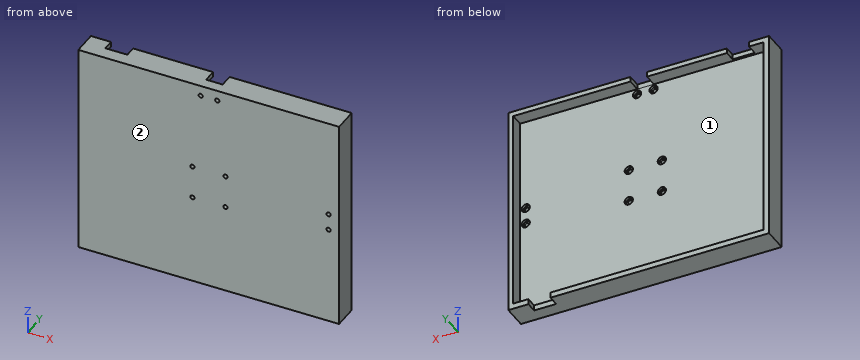
from build123d import *

# Parameters (mm, degrees)
SKETCH2_W                = 236.5
SKETCH2_H                = 193
SKETCH2_W_2              = 227
SKETCH2_H_2              = 183.5
BOSS_EXTRUDE1_DEPTH      = 12.1
SKETCH3_W                = 236.5
SKETCH3_H                = 193
BOSS_EXTRUDE2_DEPTH      = 10
SKETCH4_W                = 10
SKETCH4_H                = 10
CUT_EXTRUDE1_DEPTH       = 5
SKETCH7_W                = 20
SKETCH7_H                = 10
CUT_EXTRUDE2_DEPTH       = 5
SKETCH8_W                = 20
SKETCH8_H                = 10
CUT_EXTRUDE3_DEPTH       = 5
SKETCH32_W               = 20
SKETCH32_H               = 12.1
CUT_EXTRUDE14_DEPTH      = 6
SKETCH34_R               = 1.925
CUT_EXTRUDE16_DEPTH      = 11
SKETCH35_R               = 3.75
SKETCH35_R_2             = 1.925
CUT_EXTRUDE17_DEPTH      = 2.4
SKETCH36_W               = 20
SKETCH36_H               = 12.1
BOSS_EXTRUDE9_DEPTH      = 5
SKETCH37_W               = 15
SKETCH37_H               = 12.1
CUT_EXTRUDE18_DEPTH      = 5
SKETCH44_R               = 1.925
CUT_EXTRUDE21_DEPTH      = 13.1
CUT_EXTRUDE21_DEPTH_BACK = 11
SKETCH44_4_R             = 3.75
CUT_EXTRUDE22_DEPTH      = 2.5
SKETCH47_R               = 3.75
SKETCH47_R_2             = 1.925
CUT_EXTRUDE23_DEPTH      = 2.5
SKETCH47_2_R             = 1.925
CUT_EXTRUDE24_DEPTH      = 11


with BuildPart() as part:
    # Sketch2 → Boss-Extrude1 (new body)
    with BuildSketch(Plane(origin=(0, 0, 0), x_dir=(1, 0, 0), z_dir=(0, 1, 0))):
        with Locations((113.25, -91.5)):
            Rectangle(SKETCH2_W, SKETCH2_H)
        with Locations((113.5, -91.75)):
            Rectangle(SKETCH2_W_2, SKETCH2_H_2, mode=Mode.SUBTRACT)
    extrude(amount=BOSS_EXTRUDE1_DEPTH)

    # Sketch3 → Boss-Extrude2 (add)
    with BuildSketch(Plane.XZ):
        with Locations((113.25, 91.5)):
            Rectangle(SKETCH3_W, SKETCH3_H)
    extrude(amount=BOSS_EXTRUDE2_DEPTH)

    # Sketch4 → Cut-Extrude1 (cut)
    with BuildSketch(Plane.ZY.offset(5)):
        with Locations((96.5, 7.1)):
            Rectangle(SKETCH4_W, SKETCH4_H)
        with Locations((86.5, 7.1)):
            Rectangle(SKETCH4_W, SKETCH4_H)
    extrude(amount=-CUT_EXTRUDE1_DEPTH, mode=Mode.SUBTRACT)

    # Sketch7 → Cut-Extrude2 (cut)
    with BuildSketch(Plane.XY.offset(188)):
        with Locations((23.25, 7.1)):
            Rectangle(SKETCH7_W, SKETCH7_H)
    extrude(amount=-CUT_EXTRUDE2_DEPTH, mode=Mode.SUBTRACT)

    # Sketch8 → Cut-Extrude3 (cut)
    with BuildSketch(Plane(origin=(0, 0, -5), x_dir=(-1, 0, 0), z_dir=(0, 0, -1))):
        with Locations((-203.25, 7.1)):
            Rectangle(SKETCH8_W, SKETCH8_H)
    extrude(amount=-CUT_EXTRUDE3_DEPTH, mode=Mode.SUBTRACT)

    # Sketch32 → Cut-Extrude14 (cut, through all)
    with BuildSketch(Plane(origin=(0, 0, 0), x_dir=(0, 0, -1), z_dir=(1, 0, 0))):
        with Locations((-91.5, 6.05)):
            Rectangle(SKETCH32_W, SKETCH32_H)
    extrude(amount=-CUT_EXTRUDE14_DEPTH, mode=Mode.SUBTRACT)

    # Sketch34 → Cut-Extrude16 (cut, through all)
    with BuildSketch(Plane(origin=(0, 0, 0), x_dir=(1, 0, 0), z_dir=(0, 1, 0))):
        with Locations((128.5, -76.64384905)):
            Circle(SKETCH34_R)
        with Locations((128.467672433, -106.643831632)):
            Circle(SKETCH34_R)
        with Locations((98.532327567, -106.643831632)):
            Circle(SKETCH34_R)
        with Locations((98.5, -76.64384905)):
            Circle(SKETCH34_R)
    extrude(amount=-CUT_EXTRUDE16_DEPTH, mode=Mode.SUBTRACT)

    # Sketch35 → Cut-Extrude17 (cut)
    with BuildSketch(Plane(origin=(0, 0, 0), x_dir=(1, 0, 0), z_dir=(0, 1, 0))):
        with Locations((98.5, -76.64384905)):
            Circle(SKETCH35_R)
        with Locations((98.5, -76.64384905)):
            Circle(SKETCH35_R_2, mode=Mode.SUBTRACT)
        with Locations((128.5, -76.64384905)):
            Circle(SKETCH35_R)
        with Locations((128.5, -76.64384905)):
            Circle(SKETCH35_R_2, mode=Mode.SUBTRACT)
        with Locations((98.532327567, -106.643831632)):
            Circle(SKETCH35_R)
        with Locations((98.532327567, -106.643831632)):
            Circle(SKETCH35_R_2, mode=Mode.SUBTRACT)
        with Locations((128.467672433, -106.643831632)):
            Circle(SKETCH35_R)
    extrude(amount=-CUT_EXTRUDE17_DEPTH, mode=Mode.SUBTRACT)

    # Sketch36 → Boss-Extrude9 (add)
    with BuildSketch(Plane(origin=(0, 0, 0), x_dir=(0, 0, -1), z_dir=(1, 0, 0))):
        with Locations((-91.5, 6.05)):
            Rectangle(SKETCH36_W, SKETCH36_H)
    extrude(amount=-BOSS_EXTRUDE9_DEPTH)

    # Sketch37 → Cut-Extrude18 (cut)
    with BuildSketch(Plane.XY.offset(188)):
        with Locations((113.25, 6.0501)):
            Rectangle(SKETCH37_W, SKETCH37_H)
    extrude(amount=-CUT_EXTRUDE18_DEPTH, mode=Mode.SUBTRACT)

    # Sketch44 → Cut-Extrude21 (cut, two sides)
    with BuildSketch(Plane(origin=(0, 0, 0), x_dir=(1, 0, 0), z_dir=(0, 1, 0))) as cut_extrude21_sk:
        with Locations((121, -178.5)):
            Circle(SKETCH44_R)
        with Locations((106, -178.5)):
            Circle(SKETCH44_R)
    extrude(amount=CUT_EXTRUDE21_DEPTH, mode=Mode.SUBTRACT)
    extrude(cut_extrude21_sk.sketch, amount=-CUT_EXTRUDE21_DEPTH_BACK, mode=Mode.SUBTRACT)

    # Sketch44<4> → Cut-Extrude22 (cut)
    with BuildSketch(Plane(origin=(0, 0, 0), x_dir=(1, 0, 0), z_dir=(0, 1, 0))):
        with Locations((121, -178.5)):
            Circle(SKETCH44_4_R)
        with Locations((106, -178.5)):
            Circle(SKETCH44_4_R)
    extrude(amount=-CUT_EXTRUDE22_DEPTH, mode=Mode.SUBTRACT)

    # Sketch47 → Cut-Extrude23 (cut)
    with BuildSketch(Plane(origin=(0, 0, 0), x_dir=(1, 0, 0), z_dir=(0, 1, 0))):
        with Locations((222, -84.25)):
            Circle(SKETCH47_R)
        with Locations((222, -84.25)):
            Circle(SKETCH47_R_2, mode=Mode.SUBTRACT)
        with Locations((222, -99.25)):
            Circle(SKETCH47_R)
        with Locations((222, -99.25)):
            Circle(SKETCH47_R_2, mode=Mode.SUBTRACT)
    extrude(amount=-CUT_EXTRUDE23_DEPTH, mode=Mode.SUBTRACT)

    # Sketch47<2> → Cut-Extrude24 (cut, through all)
    with BuildSketch(Plane(origin=(0, 0, 0), x_dir=(1, 0, 0), z_dir=(0, 1, 0))):
        with Locations((222, -84.25)):
            Circle(SKETCH47_2_R)
        with Locations((222, -99.25)):
            Circle(SKETCH47_2_R)
    extrude(amount=-CUT_EXTRUDE24_DEPTH, mode=Mode.SUBTRACT)


solid = part.part
Can you work these out from the model? Positions are in its coordinate system, mm. Face numbers are marked on the shaded views. Give positions to 0.01 mm unless a question says otherwise; leave off trailing zeros. Order: outer loops, then holes, each group sorted by start corner. A loop starts at its lowest first (then second) coordinate and runs counter-clockwise, first axis right, second up. Notation, with made-up numbers: M 6,-4 L 60,-4 A32 ccw 60,22 Z; hole C 78.25,77 d6. An arc over 180 degrees is marked long. Use a Markdown table: item, result. Add a question column.
Item 1: Suppose I cut it at B-B (x = 138). List the corners of the cut face in (y, z) for me, then the cut area to 3 significant figures.
Item 2: Suppose I cut it at A-A (z = 62.5). List the corners of the cut face in (x, y) for me.
Item 3: We'd pull the mould along X, two halves only. Please class the marked faces 1 and 2: +X half, -X half, draft (parallel to the pull), parting line (faces both ways), or undercut.
Item 4: Will these pins go through, and if not, where does the flat tip stop? pin 1 (8.5 mm diameter, centred on x = 98.5, z = 76.64, fed in from +Y); pin 2 (6 mm diameter, centred on x = 98.5, z = 76.64, fed in from +Y).
Item 5: If I drill on L1, parallel to Z at x = 128.5, y = -1.8; L2, parallel to X at y = -0.5, z = 107; L3, parallel to X at y = 1.5, z = 158, over which ranges is the centre line in solid material (lowest first)? Write a range as [from, to].
Answer sheet:
| question | item | result |
|---|---|---|
| 1 | outline | M -10,-5 L 12.1,-5 L 12.1,0 L 0,0 L 0,183.5 L 12.1,183.5 L 12.1,188 L -10,188 Z |
| 1 | area | 2,040 mm² |
| 2 | outline | M -5,-10 L 231.5,-10 L 231.5,12.1 L 227,12.1 L 227,0 L 0,0 L 0,12.1 L -5,12.1 Z |
| 3 | face 1 | undercut |
| 3 | face 2 | draft |
| 4 | pin 1 | stops at y = 0 |
| 4 | pin 2 | stops at y = -2.4 |
| 5 | L1 | z = [-5, 72.89], [80.39, 102.89], [110.39, 188] |
| 5 | L2 | x = [-5, 94.8], [102.27, 124.73], [132.2, 231.5] |
| 5 | L3 | x = [-5, 0], [227, 231.5] |
